Input: dimensioned drawing with shaded views. Units: mm. Origin: part minimum x, y, z. A direction names the side the tool comes from. Coordinates: 2 decimals unless noted, no trailing zeros. Loops run counter-clockwise (first coordinate to the right, second up) from the corner with the lowest first, then second, coordinate; pieces in that order, holes last. Notation, with made-up numbers: (17.5, 16) - (54.5, 16) arc R25 ccw to (54.5, 37) - close; hole circle Ø10 at (-8, 58). An arc over 180 degrees is marked (long way). Put each result on its own line as item: value. Start each with the question number.
1) Section C-C on z = 8.5. Output: boundary loops of the cut face in (x, y).
2) Reachability of the marked faces 1, 2, 3 and 4 from +Z, -Z, +X, -X, +Y, -Y: full face, straight path, thin tool, end or side. Return the list, or none.
3) Section D-D on x = 10.25. Output: boundary loops of the cut face in (y, z).
4) Section B-B on y = 7.5. Output: boundary loops of the cut face in (x, z).
5) Section A-A on x = 7.5. Output: boundary loops of the cut face in (y, z).
6) Material intervals for line 1 along Y through (x, z) = (7.5, 7.75); line 2 along Y through (x, z) = (7.5, 4.75); line 3 along X through (y, z) = (7.5, 6.5), sorted ascending. Write a range as from..to.
7) Contact query for flat-ended pins moving along their axis: pin 1 Ø3 at (x, z) = (4, 4.5) entering from -Y; pin 2 Ø1 at (y, z) = (10.5, 5.5) entering from -X; pin 3 Ø1 at (x, y) = (4.5, 12) entering from +Z; pin 4 Ø4 at (x, y) = (6, 3) entering from -Z. Output: stop coordinate, or through.
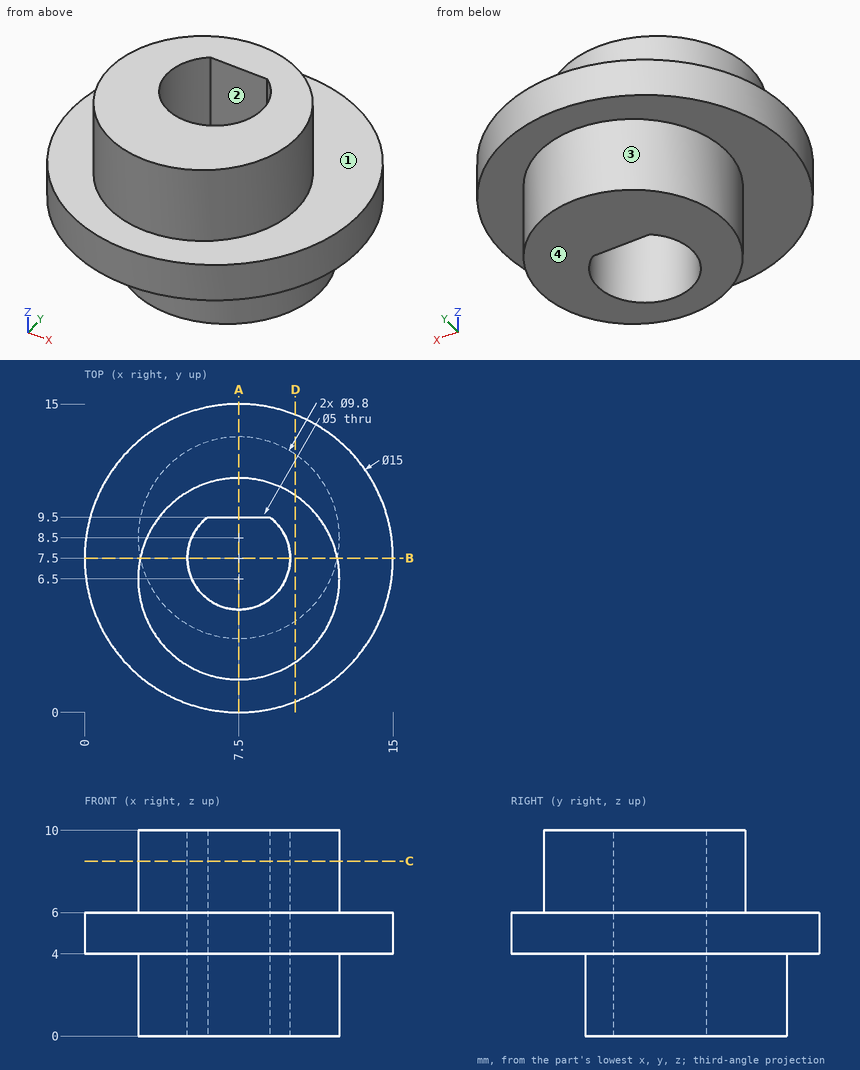
Answer block:
1. outline: circle Ø9.8 at (7.5, 6.5); hole (6, 9.5) arc R2.5 ccw (long way) to (9, 9.5) - close
2. face 1: +Z
2. face 2: +Z, -Z
2. face 3: -Z
2. face 4: -Z, +X, -X, +Y, -Y
3. outline: (0.52, 4) - (4.44, 4) - (4.44, 0) - (12.56, 0) - (12.56, 4) - (14.48, 4) - (14.48, 6) - (10.56, 6) - (10.56, 10) - (2.44, 10) - (2.44, 6) - (0.52, 6) - close
4. outline: (0, 4) - (2.7, 4) - (2.7, 0) - (5, 0) - (5, 10) - (2.7, 10) - (2.7, 6) - (0, 6) - close; (10, 0) - (12.3, 0) - (12.3, 4) - (15, 4) - (15, 6) - (12.3, 6) - (12.3, 10) - (10, 10) - close
5. outline: (0, 4) - (3.6, 4) - (3.6, 0) - (5, 0) - (5, 10) - (1.6, 10) - (1.6, 6) - (0, 6) - close; (9.5, 0) - (13.4, 0) - (13.4, 4) - (15, 4) - (15, 6) - (11.4, 6) - (11.4, 10) - (9.5, 10) - close
6. line 1: y = 1.6..5, 9.5..11.4
6. line 2: y = 0..5, 9.5..15
6. line 3: x = 2.7..5, 10..12.3
7. pin 1: stops at y = 0.27
7. pin 2: stops at x = 0.43
7. pin 3: stops at z = 6
7. pin 4: stops at z = 0
